Here's how the part is built. I have some questions about the finished solid (model axes, mm). Face numbers are marked on the shaded views. A direction names the side the tool comes from. Coordinates: 2 decimals unless noted, no trailing zeros. Write each loop counter-clockwise with the first axis right and the second up, starting at its lowest first coordinate (ties: lowest second). Pieces come first, ordered by that corner, then holes.
Item 1: I'm going to push flat-ended pins straight in: pin 1 Ø8 at (x, z) = (-9, 17.5) entering from -Y; pin 2 Ø4 at (x, y) = (27, -12) entering from +Z; pin 3 Ø10 at (x, z) = (17, 2.5) entering from -Y. Where does each tip first touch, or does it pass through?
Item 2: If we section it at A-A (y = 0): Please give me the cut outline in (x, z) (3 decimals).
Item 3: For the marked faces 1, 2, 3 and 4, which set-ups out of +Z, -Z, +X, -X, +Y, -Y let a thin tool reach every point of the face, with its end or its side?
Item 4: We'd pull the mould along Y, two halves only. Please class the marked faces 5, 6 and 7: +Y half, -Y half, draft (parallel to the pull), parting line (faces both ways), or undercut.
Item 5: If I drill on line 1 (Z direction, x = -19, y = 17.5) (3 decimals); line 2 (Y direction, x = 0, z = 18) (3 decimals); line 3 (Y direction, x = -5, z = 55), over which ranges is the centre line in solid material (lowest first)?
Item 6: If we section it at D-D (y = 44): Please give me the cut outline in (x, z) (3 decimals), then the cut area to 3 significant figures.
Item 7: If we section it at C-C (z = 21): Please give me the cut outline in (x, y) (3 decimals).
from build123d import *

# Parameters (mm, degrees)
SKETCH1_R           = 50.8
BOSS_EXTRUDE1_DEPTH = 3.175
SKETCH3_R           = 25.4
BOSS_EXTRUDE2_DEPTH = 59.055
SKETCH4_R           = 50.8
BOSS_EXTRUDE3_DEPTH = 3.175
SKETCH5_R           = 19.05
BOSS_EXTRUDE4_DEPTH = 12.7
SKETCH6_R           = 19.05
BOSS_EXTRUDE5_DEPTH = 12.7
SKETCH7_R           = 9.525
CUT_EXTRUDE1_DEPTH  = 88.63


with BuildPart() as part:
    # Sketch1 → Boss-Extrude1 (new body)
    with BuildSketch(Plane.XY):
        Circle(SKETCH1_R)
    extrude(amount=BOSS_EXTRUDE1_DEPTH)

    # Sketch3 → Boss-Extrude2 (add)
    with BuildSketch(Plane.XY):
        Circle(SKETCH3_R)
    extrude(amount=BOSS_EXTRUDE2_DEPTH)

    # Sketch4 → Boss-Extrude3 (add)
    with BuildSketch(Plane.XY.offset(59.055)):
        Circle(SKETCH4_R)
    extrude(amount=BOSS_EXTRUDE3_DEPTH)

    # Sketch5 → Boss-Extrude4 (add)
    with BuildSketch(Plane.XY.offset(62.23)):
        Circle(SKETCH5_R)
    extrude(amount=BOSS_EXTRUDE4_DEPTH)

    # Sketch6 → Boss-Extrude5 (add)
    with BuildSketch(Plane(origin=(0, 0, 0), x_dir=(-1, 0, 0), z_dir=(0, 0, -1))):
        Circle(SKETCH6_R)
    extrude(amount=BOSS_EXTRUDE5_DEPTH)

    # Sketch7 → Cut-Extrude1 (cut, through all)
    with BuildSketch(Plane.XY.offset(74.93)):
        Circle(SKETCH7_R)
    extrude(amount=-CUT_EXTRUDE1_DEPTH, mode=Mode.SUBTRACT)


solid = part.part
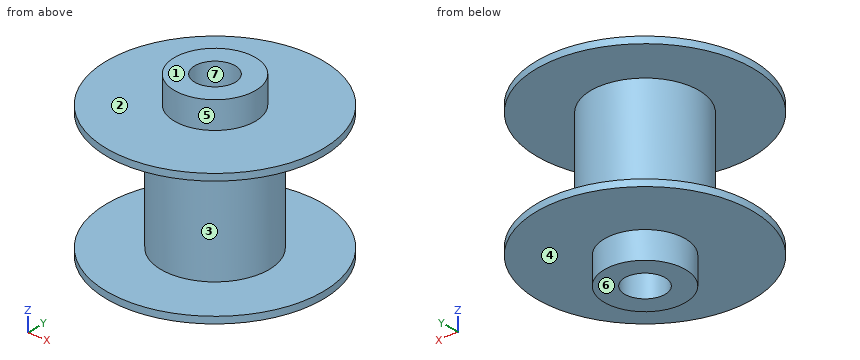
Answer list:
1. pin 1: stops at y = -24.9
1. pin 2: stops at z = 62.23
1. pin 3: stops at y = -49.36
2. outline: (-50.8, 0) - (-19.05, 0) - (-19.05, -12.7) - (-9.525, -12.7) - (-9.525, 74.93) - (-19.05, 74.93) - (-19.05, 62.23) - (-50.8, 62.23) - (-50.8, 59.055) - (-25.4, 59.055) - (-25.4, 3.175) - (-50.8, 3.175) - close; (9.525, -12.7) - (19.05, -12.7) - (19.05, 0) - (50.8, 0) - (50.8, 3.175) - (25.4, 3.175) - (25.4, 59.055) - (50.8, 59.055) - (50.8, 62.23) - (19.05, 62.23) - (19.05, 74.93) - (9.525, 74.93) - close
3. face 1: +Z, +X, -X, +Y, -Y
3. face 2: +Z
3. face 3: none
3. face 4: -Z
4. face 5: parting line
4. face 6: draft
4. face 7: undercut
5. line 1: z = 0 to 3.175, 59.055 to 62.23
5. line 2: y = -25.4 to -9.525, 9.525 to 25.4
5. line 3: y = -24.9 to -8.11, 8.11 to 24.9
6. outline: (-25.39, 0) - (25.39, 0) - (25.39, 3.175) - (-25.39, 3.175) - close; (-25.39, 59.055) - (25.39, 59.055) - (25.39, 62.23) - (-25.39, 62.23) - close
6. area: 322 mm2
7. outline: circle Ø50.8 at (0, 0); hole circle Ø19.05 at (0, 0)
